Autodesk Inventor part; units mm, degrees
ref_plane "YZ Plane" through (0, 0, 0) normal (1, 0, 0) x (0, 1, 0)
ref_plane "XZ Plane" through (0, 0, 0) normal (0, 1, 0) x (-1, 0, 0)
ref_plane "XY Plane" through (0, 0, 0) normal (0, 0, 1) x (1, 0, 0)
sketch "Эскиз1" plane through (0, 0, 0) normal (0, 0, 1) x (1, 0, 0)
  circle A0 centre (0, 0) radius 7
  circle A1 centre (0, 0) radius 6
  circle A2 centre (0, 0) radius 4.3
  line L0 (2.2504, 0) -> (3.5, 0)
  line L1 (3.5, 0) -> (-3.5, 0)
  line L2 (-3.5, -2.498) -> (-3.5, 2.498)
  line L3 (3.5, -2.498) -> (3.5, 2.498)
  line L4 (-5, 0) -> (5, 0)
  line L5 (-5, 3.3166) -> (-5, -3.3166)
  line L6 (5, -3.3166) -> (5, 3.3166)
  point P0 (-5, -3.3166)
  point P1 (5, -3.3166)
  dimension "d0" = 14
  dimension "d1" = 12
  dimension "d2" = 8.6
  dimension "d3" = 7
  dimension "d4" = 10
extrude "Выдавливание1" add sketch "Эскиз1" along normal blind 6 contours A0 | A1 L6 | L6 L4 A2 L5 A1 | A1 L5 L4 A2 L6 | L5 A1 | L4 L3 A2 | A2 L3 L4 | L4 L2 A2 | A2 L2 L4
extrude "Выдавливание2" add sketch "Эскиз1" against normal blind 1.5 contours L6 L4 A2 L5 A1 | A1 L5 L4 A2 L6 | L4 L3 A2 | A2 L3 L4 | L4 L2 A2 | A2 L2 L4
chamfer "Фаска1" distance 0.5 angle 45 4 edges at (0, 4.3, 6) (-3.5, 0, 6) (0, -4.3, 6) (3.5, 0, 6)
properties part number "ANT_INSULATOR"
Source: CAD feature listing. Evaluate the final solid. Frame: model axes, mm. A direction names the side the tool comes from. Coordinates: 2 decimals unless noted, no trailing zeros. Order: outer loops, then holes, each group sorted by start corner. A loop starts at its lowest first (then second) coordinate and runs counter-clockwise, first axis right, second up. Notation, with made-up numbers: M 46.5,34.25 L 105.5,34.25 A18 cw 105.5,47.25 Z; hole C 62,1 d10. An arc over 180 degrees is marked long. Write each question's results on one line, items separated by ' | '. Start each with the question number.
Item 1: Cut plane A-A (x = 0). Return loops of the section in (y, z), and give its area (4 significant figures).
Item 2: Set-up query: faces 5 (the face through (0, -6, -1)), 6 (the face through (0.06, 4.44, 5.64)), 7 (the face through (0.1, -4.3, 2)). Return all of +Z, -Z, +X, -X, +Y, -Y with unobstructed straight access to the full face (end or side cutting, diameter ignored); none if empty.
Item 3: Cut plane C-C (z = 1.25). Return loops of the section in (x, y), and give its area (3 significant figures).
Item 4: Line query: probe 1 along Y at (x, z) = (-1.75, 2); probe 2 along X at (y, z) = (3, -0.25); probe 3 along X at (y, z) = (-2.25, 4). Output: solid intervals per line, ascending.
Item 5: Cut plane D-D (x = 4.75). Return loops of the section in (y, z).
Item 6: Cut plane B-B (y = 0). Return loops of the section in (x, z), and give its area (4 significant figures).
Item 7: First-contact query: pin 1 Ø1.6 at (y, z) = (-0.5, -1) entering from +X; pin 2 Ø3 at (x, z) = (5, 2.5) entering from -Y; pin 3 Ø2 at (x, z) = (1.5, 4) entering from -Y. Flat tips, straight axial feed; report the tip coordinate or a pass-through.
Item 8: Draft query along Y for faces 1 (the face through (5, 0, -1)), 2 (the face through (0, 6, -1)), 3 (the face through (-3.5, 0, 2)), 4 (the face through (-0.1, 4.3, 2)). Return one class per face: pulls with the +Y half, pulls with the -Y half, needs draft (parallel to the pull), parting line crosses it, or undercut.
Checked values:
1) outline: M -7,0 L -6,0 L -6,-1.5 L -4.3,-1.5 L -4.3,5.5 L -4.8,6 L -7,6 Z; M 4.3,-1.5 L 6,-1.5 L 6,0 L 7,0 L 7,6 L 4.8,6 L 4.3,5.5 Z | area: 37.25 mm2
2) face 5: -Z, -Y | face 6: +Z | face 7: +Z, -Z
3) outline: C 0,0 d14; hole M -3.5,-2.5 A4.3 ccw 3.5,-2.5 L 3.5,2.5 A4.3 ccw -3.5,2.5 Z | area: 101 mm2
4) probe 1: y = -6.78 to -3.93, 3.93 to 6.78 | probe 2: x = -5 to -3.08, 3.08 to 5 | probe 3: x = -6.63 to -3.5, 3.5 to 6.63
5) outline: M -5.14,0 L -3.67,0 L -3.67,-1.5 L 3.67,-1.5 L 3.67,0 L 5.14,0 L 5.14,6 L -5.14,6 Z
6) outline: M -7,0 L -5,0 L -5,-1.5 L -3.5,-1.5 L -3.5,5.5 L -4,6 L -7,6 Z; M 3.5,-1.5 L 5,-1.5 L 5,0 L 7,0 L 7,6 L 4,6 L 3.5,5.5 Z | area: 46.25 mm2
7) pin 1: stops at x = 5 | pin 2: stops at y = -6.06 | pin 3: stops at y = -6.98
8) face 1: needs draft | face 2: pulls with the +Y half | face 3: undercut | face 4: undercut
